```python
from build123d import *

# Parameters (mm, degrees)
SKETCH1_R           = 2.75
SKETCH1_W           = 3
SKETCH1_H           = 5
BOSS_EXTRUDE1_DEPTH = 3
FILLET1_R           = 5


with BuildPart() as part:
    # Sketch1 → Boss-Extrude1 (new body)
    with BuildSketch(Plane(origin=(0, 0, 0), x_dir=(1, 0, 0), z_dir=(0, 1, 0))):
        Polygon((-21.821592901, -5), (-21.821592901, 10), (5.178407099, 10), (5.178407099, 5), (8.178407099, 5), (8.178407099, 0), (5.178407099, 0), (5.178407099, -5), align=None)
        with Locations((-9.121592901, 2.5)):
            Circle(SKETCH1_R, mode=Mode.SUBTRACT)
        with Locations((-16.621592901, 2.5)):
            Rectangle(SKETCH1_W, SKETCH1_H, mode=Mode.SUBTRACT)
        with Locations((-1.621592901, 2.5)):
            Rectangle(SKETCH1_W, SKETCH1_H, mode=Mode.SUBTRACT)
    extrude(amount=BOSS_EXTRUDE1_DEPTH)

    # Fillet1
    fillet1_edges = [part.edges().sort_by_distance(p)[0] for p in [
        (-21.821592901, 1.5, 5),
        (-21.821592901, 1.5, -10),
    ]]
    fillet(fillet1_edges, radius=FILLET1_R)


solid = part.part
```
Input: part model. Units: mm. Frame: model coordinates. A direction names the side the tool comes from. Give positions to 0.01 mm unless a question says otherwise; leave off trailing zeros. Order: outer loops, then holes, each group sorted by start corner. A loop starts at its lowest first (then second) coordinate and runs counter-clockwise, first axis right, second up.
1. Cut plane B-B (x = -10.25). Return loops of the section in (y, z), and give its area (3 significant figures).
Computed:
outline: (0, -10) - (3, -10) - (3, -5.01) - (0, -5.01) - close; (0, 0.01) - (3, 0.01) - (3, 5) - (0, 5) - close
area: 30.0 mm2
2. Line query: probe 1 along X at (y, z) = (1.75, -2.5); probe 2 along Z at (x, y) = (-15.25, 2.7); probe 3 along X at (y, z) = (1.5, -4.25). Output: solid intervals per line, ascending.
Computed:
probe 1: x = -21.82 to -18.12, -15.12 to -11.87, -6.37 to -3.12, -0.12 to 8.18
probe 2: z = -10 to -5, 0 to 5
probe 3: x = -21.82 to -18.12, -15.12 to -11.24, -7 to -3.12, -0.12 to 8.18
3. Cut plane D-D (z = -8). Return loops of the section in (x, y).
Computed:
outline: (-20.82, 0) - (5.18, 0) - (5.18, 3) - (-20.82, 3) - close
4. Draft query along X for faces 4 (the face through (8.178, 1, -3)), 5 (the face through (-2, 1, 0)), 6 (the face through (-6, 1, 5)), 7 (the face through (-11.304, 1.479, -0.827)). Return one class per face: released by +X, released by -X, zero draft, split by the parting line, or undercut.
Computed:
face 4: released by +X
face 5: undercut
face 6: zero draft
face 7: undercut
5. Set-up query: faces 1 (the face through (7, 1, 0)), 2 (the face through (5.178, 1, -8)), 3 (the face through (-15.122, 1, -2)). Return all of +Z, -Z, +X, -X, +Y, -Y with unobstructed straight access to the full face (end or side cutting, diameter ignored); none if empty.
Computed:
face 1: +Z, +X, +Y, -Y
face 2: -Z, +X, +Y, -Y
face 3: +Y, -Y
6. Cut plane A-A (z = -2.5). Return loops of the section in (x, y), and give its area (3 significant figures).
Computed:
outline: (-21.82, 0) - (-18.12, 0) - (-18.12, 3) - (-21.82, 3) - close; (-15.12, 0) - (-11.87, 0) - (-11.87, 3) - (-15.12, 3) - close; (-6.37, 0) - (-3.12, 0) - (-3.12, 3) - (-6.37, 3) - close; (-0.12, 0) - (8.18, 0) - (8.18, 3) - (-0.12, 3) - close
area: 55.5 mm2
7. Pin query (flat end, axial travel): pin 1 Ø1 at (y, z) = (1.5, -8) entering from +X; pin 2 Ø1.5 at (x, y) = (7, 1) entering from +Z; pin 3 Ø0.9 at (x, y) = (6, 1.5) entering from -Z. Return the tip coordinate at first contact, or that it passes through.
Computed:
pin 1: stops at x = 5.18
pin 2: stops at z = 0
pin 3: stops at z = -5
8. Cut plane C-C (y = 0.7). Return loops of the section in (x, z).
Computed:
outline: (-21.82, -5) arc R5 ccw to (-16.82, -10) - (5.18, -10) - (5.18, -5) - (8.18, -5) - (8.18, 0) - (5.18, 0) - (5.18, 5) - (-16.82, 5) arc R5 ccw to (-21.82, 0) - close; hole (-18.12, -5) - (-15.12, -5) - (-15.12, 0) - (-18.12, 0) - close; hole circle Ø5.5 at (-9.12, -2.5); hole (-3.12, -5) - (-0.12, -5) - (-0.12, 0) - (-3.12, 0) - close
